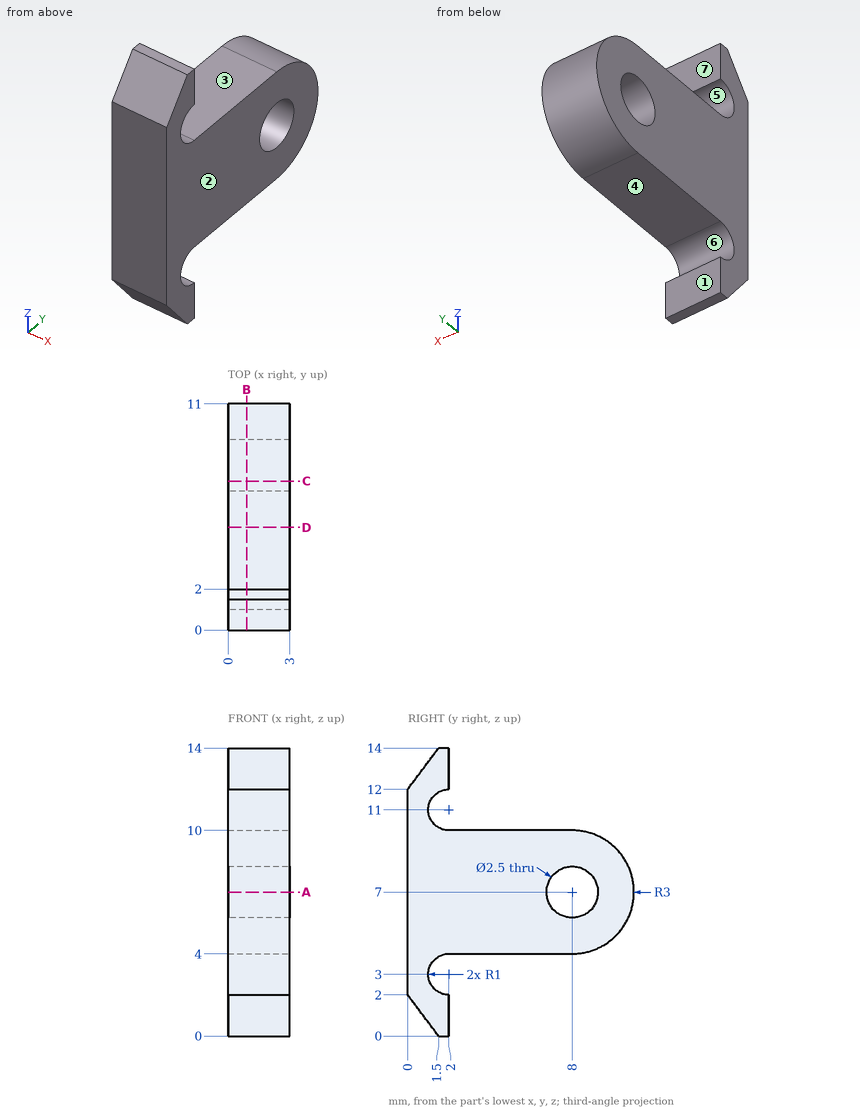
Input: dimensioned drawing with shaded views. Units: mm. Origin: part minimum x, y, z. A direction names the side the tool comes from. Round coordinates to 2 decimals unless told otherwise and drop trailing zeros. Loops run counter-clockwise (first coordinate to the right, second up) from the corner with the lowest first, then second, coordinate; pieces in that order, holes last. Notation, with made-up numbers: M 26.25,39.25 L 81.25,39.25 A20 ccw 81.25,49.25 Z; hole C -10.5,51.5 d3. An arc over 180 degrees is marked long. Answer in a Markdown table with one row per item. Add a question column.
1. Ray query, probe 1 along Y at (x, z) = (2.35, 7); probe 2 along Z at (x, y) = (1.4, 6.25); probe 3 along Y at (x, z) = (0.1, 7.5). Return the intervals inside material, ascending.
2. Mould query, pull axis Z, two halves, no side actions, for the marked faces 4, 5, 6 and 7. Classes: released by +Z, released by -Z, zero draft, split by the parting line, or undercut.
3. Section A-A (z = 7). Output: boundary loops of the cut face in (x, y).
4. Section B-B (x = 0.9). Output: boundary loops of the cut face in (y, z).
5. Section C-C (y = 7.25). Output: boundary loops of the cut face in (x, z), and give its area (3 significant figures).
6. Contact query for flat-ended pins moving along their axis: pin 1 (1.5 mm diameter, centred on y = 8, z = 7, fed in from -X); pin 2 (6 mm diameter, centred on y = 9.5, z = 9.5, fed in from -X); pin 3 (1.5 mm diameter, centred on x = 2, y = 4, fed in from +Z); pin 4 (1 mm diameter, centred on x = 1, z = 1, fed in from +Y). Output: stop coordinate, or through.
7. Section D-D (y = 5). Output: boundary loops of the cut face in (x, z).
8. Set-up query: the marked faces 1, 2 and 3. Return all of +Z, -Z, +X, -X, +Y, -Y with unobstructed straight access to the full face (end or side cutting, diameter ignored); none if empty.
Values follow:
| question | item | result |
|---|---|---|
| 1 | probe 1 | 0 to 6.75, 9.25 to 11 |
| 1 | probe 2 | 4 to 10 |
| 1 | probe 3 | 0 to 6.85, 9.15 to 10.96 |
| 2 | face 4 | released by -Z |
| 2 | face 5 | undercut |
| 2 | face 6 | undercut |
| 2 | face 7 | zero draft |
| 3 | outline | M 0,0 L 3,0 L 3,6.75 L 0,6.75 Z; M 0,9.25 L 3,9.25 L 3,11 L 0,11 Z |
| 4 | outline | M 0,2 L 1.5,0 L 2,0 L 2,2 A1 cw 2,4 L 8,4 A3 ccw 8,10 L 2,10 A1 cw 2,12 L 2,14 L 1.5,14 L 0,12 Z; hole C 8,7 d2.5 |
| 5 | outline | M 0,4 L 3,4 L 3,6 L 0,6 Z; M 0,8 L 3,8 L 3,10 L 0,10 Z |
| 5 | area | 12.0 mm^2 |
| 6 | pin 1 | through |
| 6 | pin 2 | x = 0 |
| 6 | pin 3 | z = 10 |
| 6 | pin 4 | y = 2 |
| 7 | outline | M 0,4 L 3,4 L 3,10 L 0,10 Z |
| 8 | face 1 | -Z, +X, -X, +Y |
| 8 | face 2 | +Z, -Z, +X, +Y, -Y |
| 8 | face 3 | +Z, +X, -X, +Y |
